from build123d import *

# Parameters (mm, degrees)
F0_W            = 120
F0_H            = 80
F1_DEPTH        = 2
F3_DEPTH        = 12
F5_D            = 3
F5_CBORE_D      = 5
F5_CBORE_DEPTH  = 1
F4_W            = 92.5
F4_H            = 32
F6_DEPTH        = 3
F7_W            = 10
F7_H            = 6
F8_DEPTH        = 3
F9_R            = 1
F10_R           = 3.25
F11_DEPTH       = 2
F12_R           = 1.25
F13_DEPTH       = 1
F15_D           = 3.2
F15_CBORE_D     = 5
F15_CBORE_DEPTH = 1.5


# Not quite as in the source:
# - a feature names something its author has since deleted; it is built from what else it names


with BuildPart() as f1:
    # F0 (on Top) → F1 (new body)
    with BuildSketch(Plane.XY):
        Rectangle(F0_W, F0_H)
    extrude(amount=F1_DEPTH)

    # F2 (on face) → F3 (join)
    with BuildSketch(Plane.XY.offset(2)):
        with BuildLine():
            Line((-58, 38), (-54.1715728753, 38))
            ThreePointArc((-54.1715728753, 38), (-55.2679491924, 39.4494897428), (-57, 40))
            ThreePointArc((-57, 40), (-59.1213203436, 39.1213203436), (-60, 37))
            ThreePointArc((-60, 37), (-59.4494897428, 35.2679491924), (-58, 34.1715728753))
            Line((-58, 34.1715728753), (-58, 38))
        make_face()
        with BuildLine():
            ThreePointArc((-60, 37), (-59.1213203436, 39.1213203436), (-57, 40))
            Line((-57, 40), (-60, 40))
            Line((-60, 40), (-60, 37))
        make_face()
        with BuildLine():
            ThreePointArc((-54, 37), (-54.043204321, 37.5073059362), (-54.1715728753, 38))
            Line((-54.1715728753, 38), (-58, 38))
            Line((-58, 38), (-58, 34.1715728753))
            ThreePointArc((-58, 34.1715728753), (-55.2679491924, 34.5505102572), (-54, 37))
        make_face()
        with BuildLine():
            Line((-58, -34.1715728753), (-58, 34.1715728753))
            ThreePointArc((-58, 34.1715728753), (-59.4494897428, 35.2679491924), (-60, 37))
            Line((-60, 37), (-60, -37))
            ThreePointArc((-60, -37), (-59.4494897428, -35.2679491924), (-58, -34.1715728753))
        make_face()
        with BuildLine():
            Line((-54.1715728753, 38), (54.1715728753, 38))
            ThreePointArc((54.1715728753, 38), (55.2679491924, 39.4494897428), (57, 40))
            Line((57, 40), (-57, 40))
            ThreePointArc((-57, 40), (-55.2679491924, 39.4494897428), (-54.1715728753, 38))
        make_face()
        with BuildLine():
            Line((54.1715728753, 38), (58, 38))
            Line((58, 38), (58, 34.1715728753))
            ThreePointArc((58, 34.1715728753), (59.4494897428, 35.2679491924), (60, 37))
            ThreePointArc((60, 37), (59.1213203436, 39.1213203436), (57, 40))
            ThreePointArc((57, 40), (55.2679491924, 39.4494897428), (54.1715728753, 38))
        make_face()
        with BuildLine():
            Line((58, 34.1715728753), (58, 38))
            Line((58, 38), (54.1715728753, 38))
            ThreePointArc((54.1715728753, 38), (54.8786796564, 34.8786796564), (58, 34.1715728753))
        make_face()
        with BuildLine():
            Line((60, 40), (57, 40))
            ThreePointArc((57, 40), (59.1213203436, 39.1213203436), (60, 37))
            Line((60, 37), (60, 40))
        make_face()
        with BuildLine():
            ThreePointArc((60, 37), (59.4494897428, 35.2679491924), (58, 34.1715728753))
            Line((58, 34.1715728753), (58, -34.1715728753))
            ThreePointArc((58, -34.1715728753), (59.4494897428, -35.2679491924), (60, -37))
            Line((60, -37), (60, 37))
        make_face()
        with BuildLine():
            Line((60, -40), (60, -37))
            ThreePointArc((60, -37), (59.1213203436, -39.1213203436), (57, -40))
            Line((57, -40), (60, -40))
        make_face()
        with BuildLine():
            ThreePointArc((60, -37), (59.4494897428, -35.2679491924), (58, -34.1715728753))
            Line((58, -34.1715728753), (58, -38))
            Line((58, -38), (54.1715728753, -38))
            ThreePointArc((54.1715728753, -38), (55.2679491924, -39.4494897428), (57, -40))
            ThreePointArc((57, -40), (59.1213203436, -39.1213203436), (60, -37))
        make_face()
        with BuildLine():
            Line((58, -38), (58, -34.1715728753))
            ThreePointArc((58, -34.1715728753), (54.8786796564, -34.8786796564), (54.1715728753, -38))
            Line((54.1715728753, -38), (58, -38))
        make_face()
        with BuildLine():
            ThreePointArc((57, -40), (55.2679491924, -39.4494897428), (54.1715728753, -38))
            Line((54.1715728753, -38), (-54.1715728753, -38))
            ThreePointArc((-54.1715728753, -38), (-55.2679491924, -39.4494897428), (-57, -40))
            Line((-57, -40), (57, -40))
        make_face()
        with BuildLine():
            ThreePointArc((-57, -40), (-59.1213203436, -39.1213203436), (-60, -37))
            Line((-60, -37), (-60, -40))
            Line((-60, -40), (-57, -40))
        make_face()
        with BuildLine():
            ThreePointArc((-57, -40), (-55.2679491924, -39.4494897428), (-54.1715728753, -38))
            Line((-54.1715728753, -38), (-58, -38))
            Line((-58, -38), (-58, -34.1715728753))
            ThreePointArc((-58, -34.1715728753), (-59.4494897428, -35.2679491924), (-60, -37))
            ThreePointArc((-60, -37), (-59.1213203436, -39.1213203436), (-57, -40))
        make_face()
        with BuildLine():
            Line((-58, -38), (-54.1715728753, -38))
            ThreePointArc((-54.1715728753, -38), (-54.043204321, -37.5073059362), (-54, -37))
            ThreePointArc((-54, -37), (-55.2679491924, -34.5505102572), (-58, -34.1715728753))
            Line((-58, -34.1715728753), (-58, -38))
        make_face()
    extrude(amount=-F3_DEPTH)

    # F5 (through all)
    with Locations(Plane.XY.offset(2)):
        with Locations((-54, 30), (-54, 0.8), (54.2, 0.8), (54.2, 30)):
            CounterBoreHole(F5_D / 2, F5_CBORE_D / 2, F5_CBORE_DEPTH)

    # F4 (on face) → F6 (cut)
    with BuildSketch(Plane.XY.offset(2)):
        with Locations((0.75, 15.4)):
            Rectangle(F4_W, F4_H)
    extrude(amount=-F6_DEPTH, mode=Mode.SUBTRACT)

    # F7 (on face) → F8 (cut)
    with BuildSketch(Plane.XZ.offset(40)):
        with Locations((44.2, -7)):
            Rectangle(F7_W, F7_H)
    extrude(amount=-F8_DEPTH, mode=Mode.SUBTRACT)

    # F9
    f9_edges = [f1.edges().sort_by_distance(p)[0] for p in [
        (60, -40, -4),
        (60, 40, -4),
        (-60, -40, -4),
        (-60, 40, -4),
    ]]
    fillet(f9_edges, radius=F9_R)

    # F10 (on face) → F11 (cut, through all)
    with BuildSketch(Plane.XY.offset(2)):
        with Locations((-30, -14.6378241479)):
            Circle(F10_R)
        with Locations((-30, -29.6378241479)):
            Circle(F10_R)
        with BuildLine():
            Line((-5.6, -15.8000669783), (5.6, -15.8000669783))
            ThreePointArc((5.6, -15.8000669783), (5.8828427125, -15.6829096908), (6, -15.4000669783))
            Line((6, -15.4000669783), (6, -15.0000669783))
            ThreePointArc((6, -15.0000669783), (5.8828427125, -14.7172242658), (5.6, -14.6000669783))
            Line((5.6, -14.6000669783), (-5.6, -14.6000669783))
            ThreePointArc((-5.6, -14.6000669783), (-5.8828427125, -14.7172242658), (-6, -15.0000669783))
            Line((-6, -15.0000669783), (-6, -15.4000669783))
            ThreePointArc((-6, -15.4000669783), (-5.8828427125, -15.6829096908), (-5.6, -15.8000669783))
        make_face()
        with BuildLine():
            ThreePointArc((6, -17.4000669783), (5.8828427125, -17.1172242658), (5.6, -17.0000669783))
            Line((5.6, -17.0000669783), (-5.6, -17.0000669783))
            ThreePointArc((-5.6, -17.0000669783), (-5.8828427125, -17.1172242658), (-6, -17.4000669783))
            Line((-6, -17.4000669783), (-6, -17.8000669783))
            ThreePointArc((-6, -17.8000669783), (-5.8828427125, -18.0829096908), (-5.6, -18.2000669783))
            Line((-5.6, -18.2000669783), (5.6, -18.2000669783))
            ThreePointArc((5.6, -18.2000669783), (5.8828427125, -18.0829096908), (6, -17.8000669783))
            Line((6, -17.8000669783), (6, -17.4000669783))
        make_face()
        with BuildLine():
            ThreePointArc((6, -19.8000669783), (5.8828427125, -19.5172242658), (5.6, -19.4000669783))
            Line((5.6, -19.4000669783), (-5.6, -19.4000669783))
            ThreePointArc((-5.6, -19.4000669783), (-5.8828427125, -19.5172242658), (-6, -19.8000669783))
            Line((-6, -19.8000669783), (-6, -20.2000669783))
            ThreePointArc((-6, -20.2000669783), (-5.8828427125, -20.4829096908), (-5.6, -20.6000669783))
            Line((-5.6, -20.6000669783), (5.6, -20.6000669783))
            ThreePointArc((5.6, -20.6000669783), (5.8828427125, -20.4829096908), (6, -20.2000669783))
            Line((6, -20.2000669783), (6, -19.8000669783))
        make_face()
        with BuildLine():
            ThreePointArc((6, -22.2000669783), (5.8828427125, -21.9172242658), (5.6, -21.8000669783))
            Line((5.6, -21.8000669783), (-5.6, -21.8000669783))
            ThreePointArc((-5.6, -21.8000669783), (-5.8828427125, -21.9172242658), (-6, -22.2000669783))
            Line((-6, -22.2000669783), (-6, -22.6000669783))
            ThreePointArc((-6, -22.6000669783), (-5.8828427125, -22.8829096908), (-5.6, -23.0000669783))
            Line((-5.6, -23.0000669783), (5.6, -23.0000669783))
            ThreePointArc((5.6, -23.0000669783), (5.8828427125, -22.8829096908), (6, -22.6000669783))
            Line((6, -22.6000669783), (6, -22.2000669783))
        make_face()
        with BuildLine():
            ThreePointArc((6, -24.6000669783), (5.8828427125, -24.3172242658), (5.6, -24.2000669783))
            Line((5.6, -24.2000669783), (-5.6, -24.2000669783))
            ThreePointArc((-5.6, -24.2000669783), (-5.8828427125, -24.3172242658), (-6, -24.6000669783))
            Line((-6, -24.6000669783), (-6, -25.0000669783))
            ThreePointArc((-6, -25.0000669783), (-5.8828427125, -25.2829096908), (-5.6, -25.4000669783))
            Line((-5.6, -25.4000669783), (5.6, -25.4000669783))
            ThreePointArc((5.6, -25.4000669783), (5.8828427125, -25.2829096908), (6, -25.0000669783))
            Line((6, -25.0000669783), (6, -24.6000669783))
        make_face()
    extrude(amount=-F11_DEPTH, mode=Mode.SUBTRACT)

    # F12 (on face) → F13 (cut)
    with BuildSketch(Plane(origin=(0, 0, 0), x_dir=(1, 0, 0), z_dir=(0, 0, -1))):
        with Locations((17.5, 20.0000669783)):
            Circle(F12_R)
        with Locations((-17.5, 20.0000669783)):
            Circle(F12_R)
    extrude(amount=-F13_DEPTH, mode=Mode.SUBTRACT)

    # F15 (through all)
    with Locations(Plane.XY.offset(2)):
        with Locations((-57, 37), (57, 37), (57, -37), (-57, -37)):
            CounterBoreHole(F15_D / 2, F15_CBORE_D / 2, F15_CBORE_DEPTH)


solid = f1.part
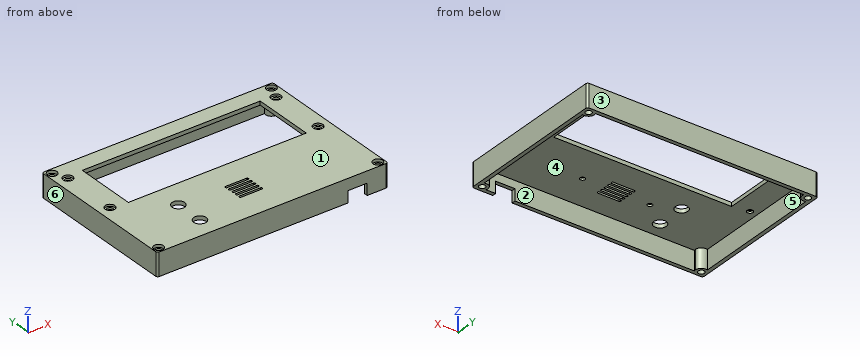
The model under review builds one solid part; all positions refer to its coordinate system, in mm. Face numbers are marked on the shaded views. A direction names the side the tool comes from. Round coordinates to 2 decimals unless told otherwise and drop trailing zeros. Loops run counter-clockwise (first coordinate to the right, second up) from the corner with the lowest first, then second, coordinate; pieces in that order, holes last. Notation, with made-up numbers: M 23,15.5 L 39,15.5 A18 ccw 39,37.5 Z; hole C 89,9.25 d9. An arc over 180 degrees is marked long. Answer as CSV lines item,"result".
1. We need section B-B (z = -8.75). Give the boundary of the cut face in (x, y), plus the area to 3 significant figures.
Outcome:
outline,"M -60,-39 A1 ccw -59,-40 L 39.2,-40 L 39.2,-38 L -54.17,-38 A3 ccw -58,-34.17 L -58,34.17 A3 ccw -54.17,38 L 54.17,38 A3 ccw 58,34.17 L 58,-34.17 A3 ccw 54.17,-38 L 49.2,-38 L 49.2,-40 L 59,-40 A1 ccw 60,-39 L 60,39 A1 ccw 59,40 L -59,40 A1 ccw -60,39 Z; hole C -57,-37 d3.2; hole C -57,37 d3.2; hole C 57,-37 d3.2; hole C 57,37 d3.2"
area,"787 mm2"
2. We need section D-D (x = -30). Give the boundary of the cut face in (y, z), plus the area to 3 significant figures.
Outcome:
outline,"M -40,-10 L -38,-10 L -38,0 L -32.89,0 L -32.89,2 L -40,2 Z; M -26.39,0 L -17.89,0 L -17.89,2 L -26.39,2 Z; M -11.39,0 L -0.6,0 L -0.6,2 L -11.39,2 Z; M 31.4,0 L 38,0 L 38,-10 L 40,-10 L 40,2 L 31.4,2 Z"
area,"110 mm2"
3. We need section C-C (y = 20). Give the boundary of the cut face in (x, z), plus the area to 3 significant figures.
Outcome:
outline,"M -60,-10 L -58,-10 L -58,0 L -45.5,0 L -45.5,2 L -60,2 Z; M 47,0 L 58,0 L 58,-10 L 60,-10 L 60,2 L 47,2 Z"
area,"95.0 mm2"
4. For the marked faces 5 and 6, list the 3-axis set-ups (+Z, -Z, +X, -X, +Y, -Y) from which the entire face can be reached by the end or side of a thin tool; tool diameter is ignored.
Outcome:
face 5,"-Z"
face 6,"+Z, -Z, -X, +Y, -Y"
5. Insertion check: pin 1 Ø2.5 at (x, y) = (-54.5, 1.5) entering from +Z; pin 2 Ø1.8 at (x, y) = (54.2, 0.8) entering from +Z; pin 3 Ø1.5 at (x, y) = (56.5, -36) entering from +Z. Each pin has a flat end and moves straight along its axis. Give the tip position at first contact, or say it passes through.
Outcome:
pin 1,"stops at z = 1"
pin 2,"passes through"
pin 3,"stops at z = 0.5"
6. To check wall thickness, follow L1, parallel to Y at x = 57, z = -1.5; L2, parallel to Y at x = -21.5, z = -6.5; L3, parallel to X at y = 36, z = -3.5. State the ranges of each line that lie inside material, in increasing order. Write a range as [from, to].
Outcome:
L1,"y = [-40, -38.6], [-35.4, -34], [34, 35.4], [38.6, 40]"
L2,"y = [-40, -38], [38, 40]"
L3,"x = [-60, -58.25], [-55.75, -54.17], [54.17, 55.75], [58.25, 60]"
7. Draft analysis for pull direction Y (two halves, no side actions). For the marked faces 1, 2, 3 and 4, state which applies: pulls with the +Y half, pulls with the -Y half, needs draft (parallel to the pull), parting line crosses it, or undercut.
Outcome:
face 1,"needs draft"
face 2,"undercut"
face 3,"pulls with the +Y half"
face 4,"undercut"
8. We need section A-A (x = 43.5). Give the boundary of the cut face in (y, z), plus the area to 3 significant figures.
Outcome:
outline,"M -40,-4 L -38,-4 L -38,0 L -0.6,0 L -0.6,2 L -40,2 Z; M 31.4,0 L 38,0 L 38,-10 L 40,-10 L 40,2 L 31.4,2 Z"
area,"124 mm2"
